Read the model definition and answer for the solid it produces. Units are mm, in the model's axes. A direction names the side the tool comes from. Round coordinates to 2 decimals unless told otherwise and drop trailing zeros. Order: outer loops, then holes, each group sorted by start corner. A loop starts at its lowest first (then second) coordinate and runs counter-clockwise, first axis right, second up. Notation, with made-up numbers: M 27.25,6.25 L 33.25,6.25 A30 cw 33.25,41.25 Z; hole C 47,81.5 d10. An arc over 180 degrees is marked long. Use one line per item in the form item = value. Start each with the question number.
Autodesk Inventor part; units mm, degrees
ref_plane "YZ Plane" through (0, 0, 0) normal (1, 0, 0) x (0, 1, 0)
ref_plane "XZ Plane" through (0, 0, 0) normal (0, 1, 0) x (-1, 0, 0)
ref_plane "XY Plane" through (0, 0, 0) normal (0, 0, 1) x (1, 0, 0)
sketch "Boceto1" plane through (0, 0, 0) normal (1, 0, 0) x (0, 1, 0)
  circle A0 centre (0, 0) radius 25
  dimension "d9" = 50
extrude "Extrusión1" add sketch "Boceto1" along normal blind 8
sketch "Boceto2" plane through (0, 0, 0) normal (-1, 0, 0) x (0, 0, 1)
  circle A0 centre (0, 0) radius 25
hole "Agujero1" at (0, 0, 0) direction (1, 0, 0) diameter 31.3762 end through all
chamfer "Chaflán1" distance 1 angle 45 4 edges at (0, -25, 0) (8, -25, 0) (0, 0, -15.6881) (8, 0, -15.6881)
sketch "Boceto3" plane through (0, 0, 0) normal (-1, 0, 0) x (0, 0, 1)
  circle A0 centre (0, 0) radius 24
  circle A1 centre (0, 0) radius 25
  line L0 (3, -25) -> (-3, -25)
  line L1 (-3, -25) -> (-3, -22)
  line L2 (-3, -22) -> (3, -22)
  line L3 (3, -22) -> (3, -25)
  point P0 (0, -22)
  dimension "d13" = 6
  dimension "d14" = 3
extrude "Extrusión2" cut sketch "Boceto3" against normal through all contours L1 L2 L3 A0 | A0 L3 A1 L1 | A1 L0 L1 | L3 L0 A1 picked at (-0.3341, -22.6597) picked at (0, -24.3194)
fillet "Empalme1" radius 0.5 2 edges at (4, -22, -3) (4, -22, 3)
pattern_circular "Patrón circular1" count 4 over 360 about axis through (71.1618, 0, 0) along (-1, 0, 0) of "Extrusión2", "Empalme1"
properties part number "retenedor_plato"
Item 1: Section C-C (x = 5.75) is taken. Write down the section's boundary in (y, z).
Item 2: Given P1, Ø1.9, axis at x = 5.5, z = 23.5, coming from the -Y side; P2, Ø12, axis at y = 7, z = 7.5, coming from the +X side; P3, Ø2.5, axis at x = 6, z = -24, coming from the -Y side, each flat-ended and moving along its own axis, determine where each tip first touches the part or whether it passes through.
Item 3: Section A-A (z = 0) is taken. Write down the section's boundary in (x, y).
Item 4: Find the intervals of material crossed by L1, parallel to Y at x = 3.75, z = 0; L2, parallel to Y at x = 2, z = 8, in increasing order. Write a range as [from, to].
Item 5: A tool of negligible diameter and unlimited length cuts with its end or side. For faces 1 (the flat face through (4, -24, 3)), 2 (the flat face through (4, 0, 22)), 3 (the flat face through (4, -3, -24)), from which of +Z, -Z, +X, -X, +Y, -Y can it reach the whole face along a straight path? Write none if from no direction.
The answers:
q1.outline = M -24.82,-3 A25 ccw -3,-24.82 L -3,-22.5 A0.5 cw -2.5,-22 L 2.5,-22 A0.5 cw 3,-22.5 L 3,-24.82 A25 ccw 24.82,-3 L 22.5,-3 A0.5 cw 22,-2.5 L 22,2.5 A0.5 cw 22.5,3 L 24.82,3 A25 ccw 3,24.82 L 3,22.5 A0.5 cw 2.5,22 L -2.5,22 A0.5 cw -3,22.5 L -3,24.82 A25 ccw -24.82,3 L -22.5,3 A0.5 cw -22,2.5 L -22,-2.5 A0.5 cw -22.5,-3 Z; hole C 0,0 d31.38
q2.P1 = -10.79
q2.P2 = 7.57
q2.P3 = -10.37
q3.outline = M 0,-22 L 8,-22 L 8,-16.69 L 7,-15.69 L 1,-15.69 L 0,-16.69 Z; M 0,16.69 L 1,15.69 L 7,15.69 L 8,16.69 L 8,22 L 0,22 Z
q4.L1 = [-22, -15.69], [15.69, 22]
q4.L2 = [-23.69, -13.5], [13.5, 23.69]
q5.face_1 = +X, -X, -Y
q5.face_2 = +Z, +X, -X
q5.face_3 = -Z, +X, -X
